Geometry: final body of the model. Coordinates: model frame, mm. Give positions to 0.01 mm unless a question says otherwise; leave off trailing zeros. Order: outer loops, then holes, each group sorted by start corner. A loop starts at its lowest first (then second) coordinate and runs counter-clockwise, first axis right, second up. Notation, with made-up numbers: (47.5, -8.75) - (60.5, -8.75) arc R37 ccw to (60.5, 28.25) - close; hole circle Ø2 at (-4, -32.75). An arc over 180 degrees is marked (long way). Write item = value, one per line. Start each with the question number.
from build123d import *

# Parameters (mm, degrees)
SKETCH001_AS_DRAWN_W              = 18.720886
SKETCH001_AS_DRAWN_H              = 1.61615
EXTRUDE_DEPTH                     = 5
EXTRUDE_ONTO_SKETCH001_ROLL_ANGLE = 90
REVOLVE_ONTO_SKETCH_ROLL_ANGLE    = 90


with BuildPart() as pan_handle:
    # Sketch001 as drawn → Extrude (new)
    with BuildSketch(Plane.XY):
        with Locations((24.33337, 0.808075)):
            Rectangle(SKETCH001_AS_DRAWN_W, SKETCH001_AS_DRAWN_H)
    extrude(amount=-EXTRUDE_DEPTH)


with BuildPart() as pan_handle_1:
    # Extrude onto Sketch001 roll: moved
    add(pan_handle.part.rotate(Axis((0, 0, 0), (1, 0, 0)), EXTRUDE_ONTO_SKETCH001_ROLL_ANGLE))


with BuildPart() as pan_handle_2:
    # Extrude onto Sketch001 placement: moved
    add(pan_handle_1.part)


with BuildPart() as pan:
    # Sketch as drawn → Revolve (revolve)
    with BuildSketch(Plane.XY):
        Polygon((0, 0), (15, 0), (17.539625, 3.555642), (16.039625, 3.555642), (14.4, 1.5), (0, 1.5), align=None)
    revolve(axis=Axis((0, 0, 0), (0, 1, 0)))


with BuildPart() as pan_1:
    # Revolve onto Sketch roll: moved
    add(pan.part.rotate(Axis((0, 0, 0), (1, 0, 0)), REVOLVE_ONTO_SKETCH_ROLL_ANGLE))


with BuildPart() as pan_2:
    # Revolve onto Sketch placement: moved
    add(pan_1.part)

    # Fusion: union PAN_HANDLE
    add(pan_handle_2.part)


solid = pan_2.part
Q1. Section A-A, the plane x = 0. Return the cut outline in (y, z), then the cut area to 3 significant figures.
Q2. Pull-direction query (X, two-part tool) for faces 1 (the flat face through (0, 0, 1.5)), 2 (the flat face through (24, 2, 1.616)), 3 (the flat face through (33.694, 2, 1)); classes: +X half, -X half, draft (parallel to the pull), parting line (faces both ways), or undercut.
Q3. Contact query for flat-ended pins moving along their axis: pin 1 (2 mm diameter, centred on y = 14, z = 3, fed in from -X); pin 2 (8.5 mm diameter, centred on x = -3.5, y = -4.5, fed in from +Z); pin 3 (1.8 mm diameter, centred on x = 24, z = 1, fed in from +Y). Output: stop coordinate, or through.
Q4. Section C-C, the plane x = 25. Return the cut outline in (y, z), then the cut area to 3 significant figures.
Q5. Material intervals for line 1 along Y through (x, z) = (19.5, 0.7); line 2 along Y through (x, z) = (-1.5, 2.05); line 3 along Z through (x, y) = (11, -3), sorted ascending. Write a range as from..to.
Q6. Section B-B, the plane z = 2.75. Return the cut outline in (x, y).
The answers:
q1.outline = (-17.54, 3.56) - (-15, 0) - (15, 0) - (17.54, 3.56) - (16.04, 3.56) - (14.4, 1.5) - (-14.4, 1.5) - (-16.04, 3.56) - close
q1.area = 53.1 mm²
q2.face_1 = undercut
q2.face_2 = draft
q2.face_3 = +X half
q3.pin_1 = -11.59
q3.pin_2 = 1.5
q3.pin_3 = 5
q4.outline = (0, 0) - (5, 0) - (5, 1.62) - (0, 1.62) - close
q4.area = 8.08 mm²
q5.line_1 = 0..5
q5.line_2 = -16.4..-14.76, 14.76..16.4
q5.line_3 = 0..1.5
q6.outline = circle Ø33.93 at (0, 0); hole circle Ø30.79 at (0, 0)
